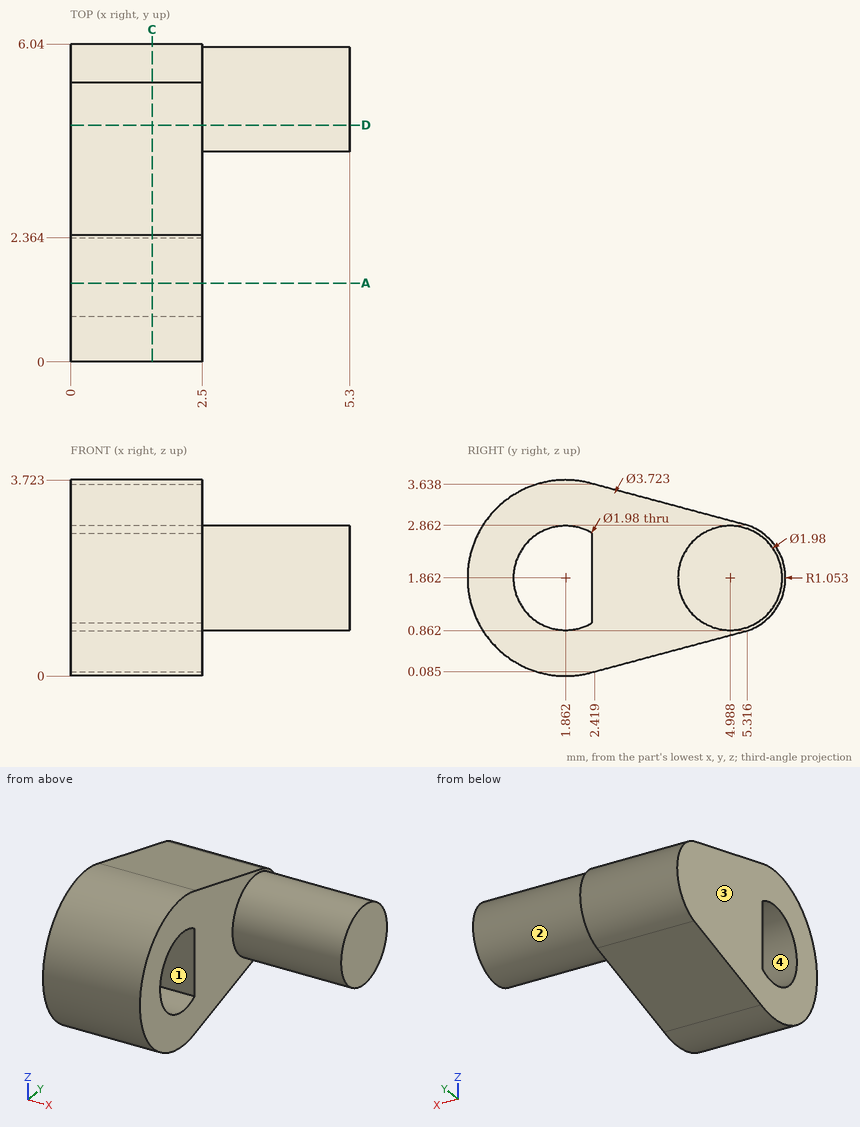
Verification items for this drawing (mm, ordinates from the low corner). Give positions to 0.01 mm unless a question says otherwise; leave off trailing zeros. Loops run counter-clockwise (first coordinate to the right, second up) from the corner with the lowest first, then second, coordinate; pieces in that order, holes last. Notation, with made-up numbers: M 61,44 L 89,44 A13 cw 89,67 Z; hole C 38.25,5 d11. An arc over 180 degrees is marked long. Write item = value, one per line. Start each with the question number.
1. Thickness scan on probe 1 along X at (y, z) = (3.5, 1.7); probe 2 along Y at (x, z) = (2.4, 2) (1 decimal); probe 3 along Z at (x, y) = (2.35, 1.5) (1 decimal). Record the ranges inside material, lowest first.
2. Draft check along Z on the marked faces 1, 2, 3 and 4. Enter one of: +Z half, -Z half, draft (parallel to the pull), parting line (faces both ways), or undercut.
3. Section check A-A, the plane y = 1.5. Enter the section's corners in (x, z) (1 decimal).
4. Go/stop test with flat-tipped pins: P1, Ø1, axis at x = 1.5, y = 2, coming from the +Z side; P2, Ø2, axis at y = 1.5, z = 1.5, coming from the +X side; P3, Ø1.5, axis at x = 4.5, y = 4.5, coming from the -Z side; P4, Ø1.5, axis at x = 4.5, y = 3, coming from the +Z side. Record where each tip stops, or that it passes through.
5. Section check C-C, the plane x = 1.55. Enter the section's corners in (y, z) (1 decimal), plus the area to 3 significant figures.
6. Section check D-D, the plane y = 4.5. Enter the section's corners in (x, z), plus the area to 3 significant figures.
Values follow:
q1.probe_1 = 0 to 2.5
q1.probe_2 = 0 to 0.9, 2.4 to 6
q1.probe_3 = 0 to 0.9, 2.8 to 3.7
q2.face_1 = undercut
q2.face_2 = parting line
q2.face_3 = draft
q2.face_4 = undercut
q3.outline = M 0,0 L 2.5,0 L 2.5,0.9 L 0,0.9 Z; M 0,2.8 L 2.5,2.8 L 2.5,3.7 L 0,3.7 Z
q4.P1 = 3.72
q4.P2 = 2.5
q4.P3 = 0.87
q4.P4 = through
q5.outline = M 2.4,0.1 L 5.3,0.9 A1.1 ccw 5.3,2.9 L 2.4,3.6 A1.9 ccw long Z; hole M 2.4,1 L 2.4,2.7 A1 ccw long Z
q5.area = 14.1 mm^2
q6.outline = M 0,0.64 L 2.5,0.64 L 2.5,1 L 5.3,1 L 5.3,2.72 L 2.5,2.72 L 2.5,3.08 L 0,3.08 Z
q6.area = 10.9 mm^2
